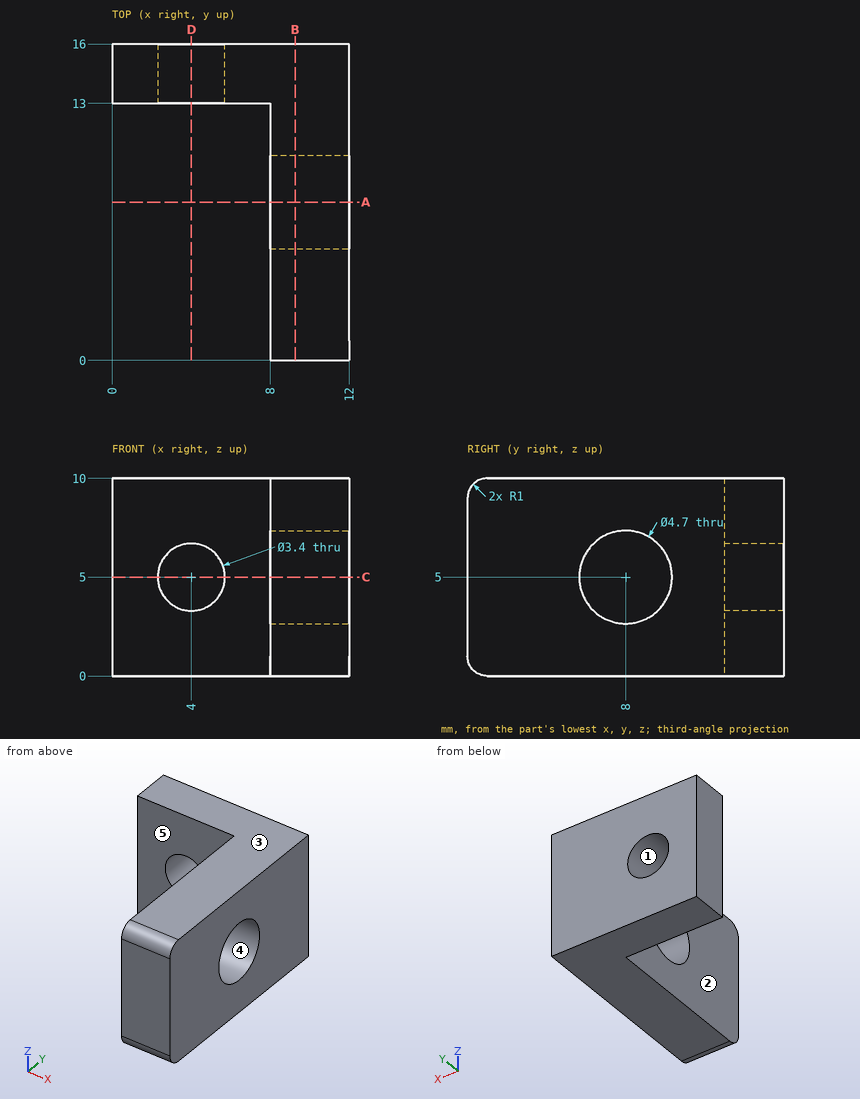
Drawing for the job (mm, zero at the part's lowest x, y, z). A direction names the side the tool comes from. Coordinates: 2 decimals unless noted, no trailing zeros. Order: outer loops, then holes, each group sorted by start corner. A loop starts at its lowest first (then second) coordinate and runs counter-clockwise, first axis right, second up. Notation, with made-up numbers: (26, -25.5) - (76, -25.5) arc R9 cw to (76, -8.5) - close; hole circle Ø1 at (10.25, 37). An arc over 180 degrees is marked (long way). Use a Markdown table: item, result. Add a question column.
(1) Which spindle directions (+Z, -Z, +X, -X, +Y, -Y) get a long thin tool onto all of the face, cutting with end or side? Do the marked faces 1 and 2. Say none if no direction does.
(2) Saw through at A-A (y = 8). Give the cut face in (x, z), then the cut area to 3 significant figures.
(3) Drill centre lines: line 1 along Z through (x, y) = (4, 13.9); line 2 along X through (y, z) = (3.5, 4.5); line 3 along Y through (x, z) = (7, 1). Where is each one in solid material? Low to high. Write a range as [from, to].
(4) Saw through at B-B (x = 9.25). Give the cut face in (y, z).
(5) Saw through at C-C (z = 5). Give the cut face in (x, y).
(6) Saw through at D-D (x = 4). Give the cut face in (y, z).
(7) Flat gauge pins, fed straight in: pin 1 (4 mm diameter, centred on y = 8, z = 5, fed in from -X); pin 2 (5 mm diameter, centred on x = 3.5, z = 7.5, fed in from -Y). Where does each tip first touch, or does it go through?
(8) Pull direction Y, two halves, no side cores. Call the marked faces 3, 4 and 5: +Y half, -Y half, draft (parallel to the pull), parting line (faces both ways), or undercut.
Solved:
| question | item | result |
|---|---|---|
| 1 | face 1 | +Y, -Y |
| 1 | face 2 | +Z, -Z, -X, -Y |
| 2 | outline | (8, 0) - (12, 0) - (12, 2.65) - (8, 2.65) - close; (8, 7.35) - (12, 7.35) - (12, 10) - (8, 10) - close |
| 2 | area | 21.2 mm² |
| 3 | line 1 | z = [0, 3.3], [6.7, 10] |
| 3 | line 2 | x = [8, 12] |
| 3 | line 3 | y = [13, 16] |
| 4 | outline | (0, 1) arc R1 ccw to (1, 0) - (16, 0) - (16, 10) - (1, 10) arc R1 ccw to (0, 9) - close; hole circle Ø4.7 at (8, 5) |
| 5 | outline | (0, 13) - (2.3, 13) - (2.3, 16) - (0, 16) - close; (5.7, 13) - (8, 13) - (8, 10.35) - (12, 10.35) - (12, 16) - (5.7, 16) - close; (8, 0) - (12, 0) - (12, 5.65) - (8, 5.65) - close |
| 6 | outline | (13, 0) - (16, 0) - (16, 3.3) - (13, 3.3) - close; (13, 6.7) - (16, 6.7) - (16, 10) - (13, 10) - close |
| 7 | pin 1 | passes through |
| 7 | pin 2 | stops at y = 13 |
| 8 | face 3 | draft |
| 8 | face 4 | undercut |
| 8 | face 5 | -Y half |
